The drawing under review shows one solid part. Ordinate dimensions are in mm from its lowest x, y, z. A direction names the side the tool comes from. Coordinates: 2 decimals unless noted, no trailing zeros. Loops run counter-clockwise (first coordinate to the right, second up) from the corner with the lowest first, then second, coordinate; pieces in that order, holes last. Notation, with made-up numbers: (49.25, 5) - (94.25, 5) arc R22 cw to (94.25, 34) - close; hole circle Ø1 at (84.25, 8). An arc over 180 degrees is marked (long way). Use one line per item in the form item = value. Start each with the question number.
1. Machinability: for the marked faces 1 and 2, which of the approach directions +Z, -Z, +X, -X, +Y, -Y give a long, thin tool a straight path to every point of the face, cutting with its end or side? Answer none if there is none.
2. Add section A-A on z = 16.5. Give the boundary of the cut face in (x, y), and give its area (3 significant figures).
3. Add section B-B on x = 47. Give the boundary of the cut face in (y, z).
4. Draft analysis for pull direction X (two halves, no side actions). For the marked faces 3, 4, 5 and 6, state which applies: +X half, -X half, draft (parallel to the pull), parting line (faces both ways), or undercut.
5. For pin 1 Ø12 at (y, z) = (98, 58) entering from -X; pin 2 Ø5 at (x, y) = (34.5, 2.5) entering from +Z; pin 3 Ø6 at (x, z) = (15, 56.5) entering from -Y; pin 4 Ø5.5 at (x, y) = (20.5, 17) entering from +Z, all flat-tipped, find the tip position at first contact; note any pin that passes through.
6. Add section C-C on y = 19. Give the boundary of the cut face in (x, z), and give its area (3 significant figures).
7. Add section D-D on x = 41. Give the boundary of the cut face in (y, z), and give its area (3 significant figures).
8. To check wall thickness, follow probe 1 along Y at (x, z) = (44, 13.5); probe 2 along Y at (x, z) = (30, 36.5); probe 3 along Z at (x, y) = (38, 67). State the ranges of each line that lie inside material, in increasing order.
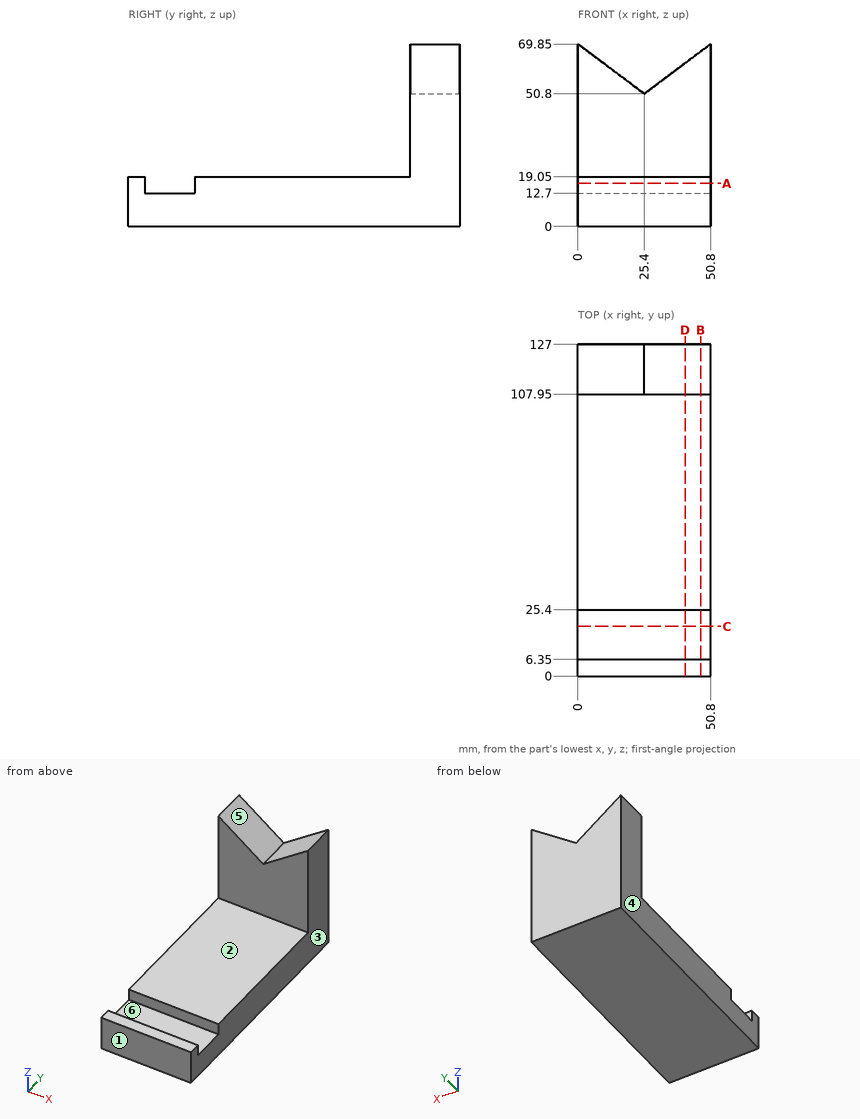
Conclusion:
q1.face_1 = +Z, -Z, +X, -X, -Y
q1.face_2 = +Z, +X, -X, -Y
q2.outline = (0, 0) - (50.8, 0) - (50.8, 6.35) - (0, 6.35) - close; (0, 25.4) - (50.8, 25.4) - (50.8, 127) - (0, 127) - close
q2.area = 5,480 mm^2
q3.outline = (0, 0) - (127, 0) - (127, 67) - (107.95, 67) - (107.95, 19.05) - (25.4, 19.05) - (25.4, 12.7) - (6.35, 12.7) - (6.35, 19.05) - (0, 19.05) - close
q4.face_3 = +X half
q4.face_4 = -X half
q4.face_5 = undercut
q4.face_6 = draft
q5.pin_1 = through
q5.pin_2 = 19.05
q5.pin_3 = 107.95
q5.pin_4 = 12.7
q6.outline = (0, 0) - (50.8, 0) - (50.8, 12.7) - (0, 12.7) - close
q6.area = 645 mm^2
q7.outline = (0, 0) - (127, 0) - (127, 62.5) - (107.95, 62.5) - (107.95, 19.05) - (25.4, 19.05) - (25.4, 12.7) - (6.35, 12.7) - (6.35, 19.05) - (0, 19.05) - close
q7.area = 3,130 mm^2
q8.probe_1 = 0 to 6.35, 25.4 to 127
q8.probe_2 = 107.95 to 127
q8.probe_3 = 0 to 19.05
